Drawing for the job (mm, zero at the part's lowest x, y, z). A direction names the side the tool comes from. Coordinates: 2 decimals unless noted, no trailing zeros. Write each loop counter-clockwise with the first axis right and the second up, starting at its lowest first coordinate (ties: lowest second). Pieces come first, ordered by that corner, then holes. Notation, with made-up numbers: (0.25, -12) -> (18.25, -12) arc R19 ccw to (18.25, 13) -> close; hole circle Ø10 at (1, -10). An arc over 180 degrees is marked (long way). Write item = value, one per line. Start each with the question number.
Q1. Pull direction X, two halves, no side cores. Call the marked faces 3, 4 and 5: released by +X, released by -X, zero draft, split by the parting line, or undercut.
Q2. Band-saw the part on D-D, the plane x = 92. List the corners of the cut face in (y, z).
Q3. Band-saw the part on C-C, the plane y = 44. List the corners of the cut face in (x, z).
Q4. Band-saw the part on A-A, the plane y = 56. List the corners of the cut face in (x, z).
Q5. Tool access for the marked faces 1 and 2: list every direction of +Z, -Z, +X, -X, +Y, -Y with a clear straight run to the whole face (end or side of a thin tool).
Q6. Pin check, flat tips, straight feed: P1, Ø4, axis at x = 35.5, y = 11.5, coming from the +Z side; P2, Ø7.5, axis at x = 56, y = 45.5, coming from the +Z side; P3, Ø6, axis at x = 28, y = 15.5, coming from the +Z side; P4, Ø5, axis at x = 25.5, y = 23, coming from the -Z side. Stop position of each tip, or through.
Q7. Probe line 1 (X direction, y = 60.5, z = 56); line 2 (Z direction, x = 49, y = 40); line 3 (Z direction, x = 64, y = 38) (1 decimal). List the from-to ranges inside material, lowest first.
Q8. Band-saw the part on B-B, the plane x = 49. List the corners of the cut face in (y, z).
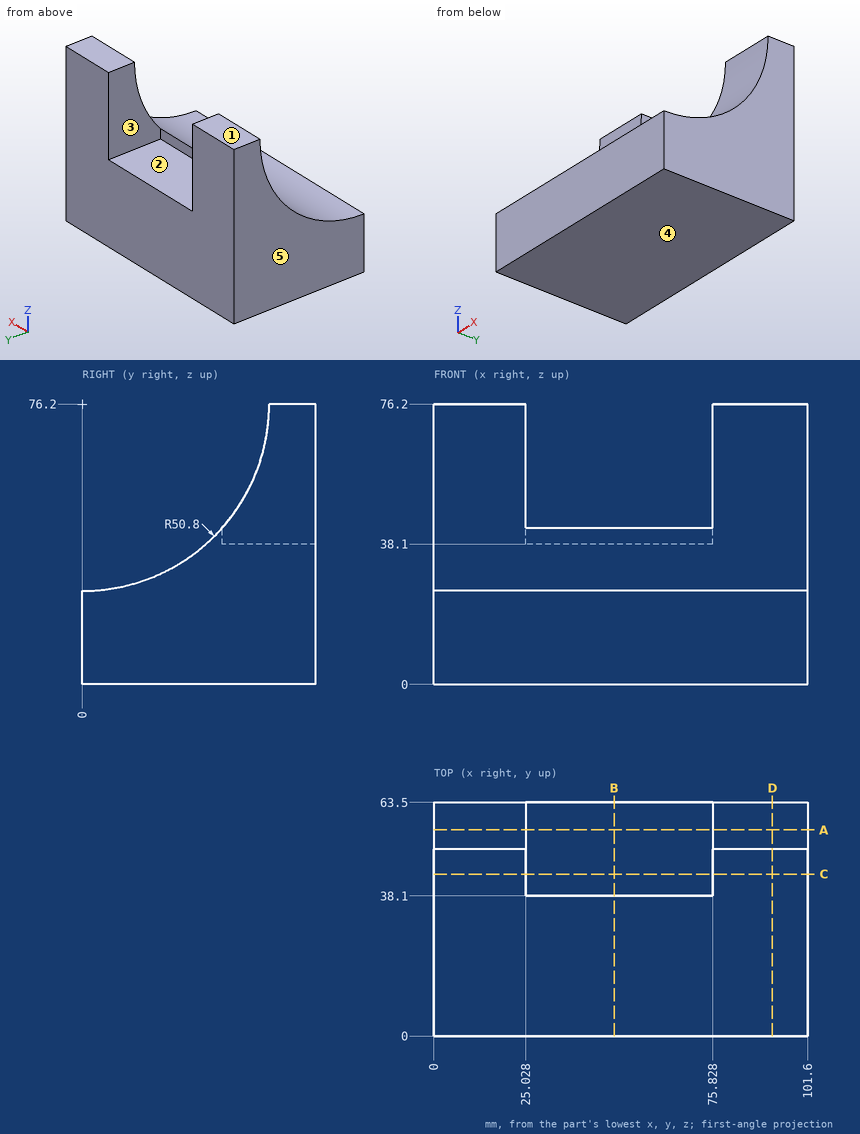
Ans:
q1.face_3 = undercut
q1.face_4 = zero draft
q1.face_5 = released by -X
q2.outline = (0, 0) -> (63.5, 0) -> (63.5, 76.2) -> (50.8, 76.2) arc R50.8 cw to (0, 25.4) -> close
q3.outline = (0, 0) -> (101.6, 0) -> (101.6, 50.81) -> (75.83, 50.81) -> (75.83, 38.1) -> (25.03, 38.1) -> (25.03, 50.81) -> (0, 50.81) -> close
q4.outline = (0, 0) -> (101.6, 0) -> (101.6, 76.2) -> (75.83, 76.2) -> (75.83, 38.1) -> (25.03, 38.1) -> (25.03, 76.2) -> (0, 76.2) -> close
q5.face_1 = +Z, +X, -X, +Y, -Y
q5.face_2 = +Z, +Y
q6.P1 = 27.23
q6.P2 = 38.1
q6.P3 = 28.89
q6.P4 = 0
q7.line_1 = 0 to 25.03, 75.83 to 101.6
q7.line_2 = 0 to 38.1
q7.line_3 = 0 to 42.5
q8.outline = (0, 0) -> (63.5, 0) -> (63.5, 38.1) -> (38.1, 38.1) -> (38.1, 42.6) arc R50.8 cw to (0, 25.4) -> close
